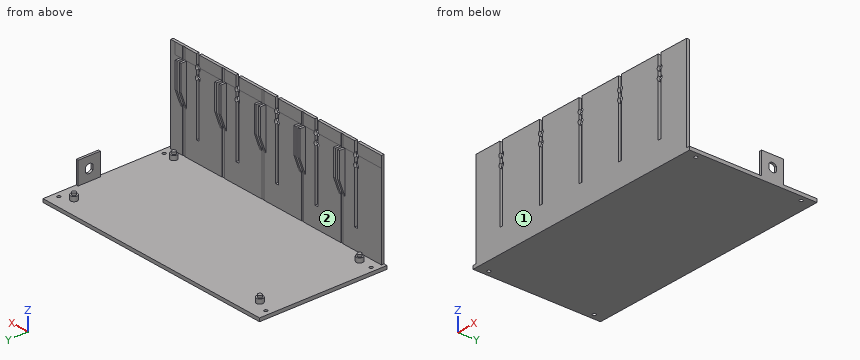
from build123d import *

# Parameters (mm, degrees)
SKETCH_W        = 226
SKETCH_H        = 115
PAD_DEPTH       = 3
PAD001_DEPTH    = 85
SKETCH002_R     = 3
PAD002_DEPTH    = 4
SKETCH003_R     = 1.75
PAD003_DEPTH    = 2
SKETCH004_R     = 1.5
POCKET_DEPTH    = 3.001
SKETCH005_W     = 3
SKETCH005_H     = 10.331698
SKETCH005_H_2   = 9.573412
SKETCH005_H_3   = 9.002111
SKETCH005_H_4   = 9.234924
SKETCH005_H_5   = 9.778156
POCKET001_DEPTH = 67
SKETCH006_R     = 2.5
POCKET002_DEPTH = 5
SKETCH008_W     = 218.676559
SKETCH008_H     = 5.389001
POCKET003_DEPTH = 10
POCKET004_DEPTH = 200
SKETCH010_W     = 2
SKETCH010_H     = 20
PAD004_DEPTH    = 20
POCKET005_DEPTH = 5
SKETCH012_W     = 3
SKETCH012_H     = 3
POCKET006_DEPTH = 85


with BuildPart() as part:
    # Sketch → Pad (new body)
    with BuildSketch(Plane.XY):
        with Locations((113, 57.5)):
            Rectangle(SKETCH_W, SKETCH_H)
    extrude(amount=PAD_DEPTH)

    # Sketch001 (on Face6 of Pad) → Pad001 (join)
    with BuildSketch(Plane.XY.offset(3)):
        Polygon((0, 0), (0, 2.4), (41.05, 2.4), (41.05, 7.4), (43.05, 7.4), (43.05, 2), (45.35, 2), (45.35, 7.4), (47.35, 7.4), (47.35, 2.4), (82.35, 2.4), (82.35, 7.4), (84.35, 7.4), (84.35, 2), (86.65, 2), (86.65, 7.4), (88.65, 7.4), (88.65, 2.4), (123.65, 2.4), (123.65, 7.4), (125.65, 7.4), (125.65, 2), (127.95, 2), (127.95, 7.4), (129.95, 7.4), (129.95, 2.4), (164.95, 2.4), (164.95, 7.4), (166.95, 7.4), (166.95, 2), (169.25, 2), (169.25, 7.4), (171.25, 7.4), (171.25, 2.4), (206.25, 2.4), (206.25, 7.4), (208.25, 7.4), (208.25, 2), (210.55, 2), (210.55, 7.4), (212.55, 7.4), (212.55, 2.4), (226, 2.4), (226, 0), align=None)
    extrude(amount=PAD001_DEPTH)

    # Sketch002 (on Face3 of Pad001) → Pad002 (join)
    with BuildSketch(Plane.XY.offset(3)):
        with Locations((17, 10)):
            Circle(SKETCH002_R)
        with Locations((17, 100)):
            Circle(SKETCH002_R)
        with Locations((211, 100)):
            Circle(SKETCH002_R)
        with Locations((211, 10)):
            Circle(SKETCH002_R)
    extrude(amount=PAD002_DEPTH)

    # Sketch003 (on Face54 of Pad002) → Pad003 (join)
    with BuildSketch(Plane.XY.offset(7)):
        with Locations((17, 100)):
            Circle(SKETCH003_R)
        with Locations((211, 100)):
            Circle(SKETCH003_R)
        with Locations((17, 10)):
            Circle(SKETCH003_R)
        with Locations((211, 10)):
            Circle(SKETCH003_R)
    extrude(amount=PAD003_DEPTH)

    # Sketch004 (on Face7 of Pad003) → Pocket (cut, through all)
    with BuildSketch(Plane.XY.offset(3)):
        with Locations((5, 105)):
            Circle(SKETCH004_R)
        with Locations((221, 105)):
            Circle(SKETCH004_R)
        with Locations((221, 10)):
            Circle(SKETCH004_R)
        with Locations((5, 10)):
            Circle(SKETCH004_R)
    extrude(amount=-POCKET_DEPTH, mode=Mode.SUBTRACT)

    # Sketch005 (on Face10 of Pocket) → Pocket001 (cut)
    with BuildSketch(Plane.XY.offset(88)):
        with Locations((29.55, 1.058323)):
            Rectangle(SKETCH005_W, SKETCH005_H)
        with Locations((70.85, 1.24642)):
            Rectangle(SKETCH005_W, SKETCH005_H_2)
        with Locations((112.15, 0.827586)):
            Rectangle(SKETCH005_W, SKETCH005_H_3)
        with Locations((153.45, 1.334431)):
            Rectangle(SKETCH005_W, SKETCH005_H_4)
        with Locations((194.75, 1.451644)):
            Rectangle(SKETCH005_W, SKETCH005_H_5)
    extrude(amount=-POCKET001_DEPTH, mode=Mode.SUBTRACT)

    # Sketch006 (on Face2 of Pocket001) → Pocket002 (cut)
    with BuildSketch(Plane.XZ):
        with Locations((29.55, 77)):
            Circle(SKETCH006_R)
        with Locations((29.55, 69)):
            Circle(SKETCH006_R)
        with Locations((70.85, 77)):
            Circle(SKETCH006_R)
        with Locations((70.85, 69)):
            Circle(SKETCH006_R)
        with Locations((112.15, 77)):
            Circle(SKETCH006_R)
        with Locations((112.15, 69)):
            Circle(SKETCH006_R)
        with Locations((153.45, 77)):
            Circle(SKETCH006_R)
        with Locations((153.45, 69)):
            Circle(SKETCH006_R)
        with Locations((194.75, 77)):
            Circle(SKETCH006_R)
        with Locations((194.75, 69)):
            Circle(SKETCH006_R)
    extrude(amount=-POCKET002_DEPTH, mode=Mode.SUBTRACT)

    # Sketch008 (on Face60 of Pocket002) → Pocket003 (cut)
    with BuildSketch(Plane.XY.offset(88)):
        with Locations((109.338279, 5.0945)):
            Rectangle(SKETCH008_W, SKETCH008_H)
    extrude(amount=-POCKET003_DEPTH, mode=Mode.SUBTRACT)

    # Sketch009 (on Face88 of Pocket003) → Pocket004 (cut)
    with BuildSketch(Plane.YZ.offset(212.55)):
        Polygon((7.4, 3), (2.4, 3), (2.4, 40.5), (7.4, 54.974999), align=None)
    extrude(amount=-POCKET004_DEPTH, mode=Mode.SUBTRACT)

    # Sketch010 (on Face132 of Pocket004) → Pad004 (join)
    with BuildSketch(Plane.XY.offset(3)):
        with Locations((225, 75)):
            Rectangle(SKETCH010_W, SKETCH010_H)
    extrude(amount=PAD004_DEPTH)

    # Sketch011 (on Face154 of Pad004) → Pocket005 (cut)
    with BuildSketch(Plane.YZ.offset(226)):
        with BuildLine():
            ThreePointArc((78.3, 15.085192), (75, 16.906731), (71.7, 15.085192))
            Line((71.7, 15.085192), (71.7, 10.92827))
            ThreePointArc((71.7, 10.92827), (75, 9.106731), (78.3, 10.92827))
            Line((78.3, 15.085192), (78.3, 10.92827))
        make_face()
    extrude(amount=-POCKET005_DEPTH, mode=Mode.SUBTRACT)

    # Sketch012 (on Face80 of Pocket005) → Pocket006 (cut)
    with BuildSketch(Plane.XY.offset(88)):
        with Locations((1.5, 1.5)):
            Rectangle(SKETCH012_W, SKETCH012_H)
        with Locations((224.5, 1.5)):
            Rectangle(SKETCH012_W, SKETCH012_H)
    extrude(amount=-POCKET006_DEPTH, mode=Mode.SUBTRACT)


solid = part.part
The listing builds one solid part. Answer for the finished solid, in the listing's coordinates (mm). Face numbers are marked on the shaded views. Coordinates: 2 decimals unless noted, no trailing zeros. Order: outer loops, then holes, each group sorted by start corner. A loop starts at its lowest first (then second) coordinate and runs counter-clockwise, first axis right, second up. Notation, with made-up numbers: M 37,58.25 L 78,58.25 A17 ccw 78,87.25 Z; hole C 79.25,30 d5. An arc over 180 degrees is marked long. Use CSV: the item, a comma, the result in double quotes.
Q1. Determine the mould class of the marked faces 1 and 2 for opening direction X: pulls with the +X half, pulls with the -X half, needs draft (parallel to the pull), parting line crosses it, or undercut.
Here are the results:
face 1,"needs draft"
face 2,"undercut"
Q2. Given pin 1 Ø0.7 at (y, z) = (1, 84) entering from -X; pin 2 Ø1.2 at (y, z) = (1.5, 74) entering from +X; pin 3 Ø1 at (x, z) = (83.5, 65) entering from +Y; pin 4 Ø4.5 at (y, z) = (5, 31.5) entering from -X, each flat-ended and moving along its own axis, determine where each tip first touches the part or whether it passes through.
Here are the results:
pin 1,"x = 3"
pin 2,"x = 223"
pin 3,"y = 7.4"
pin 4,"through"
Q3. Section C-C (y = 57) is taken. Determine the outline of the cut face in (x, z), then the cut area to 3 significant figures.
Here are the results:
outline,"M 0,0 L 226,0 L 226,3 L 0,3 Z"
area,"678 mm2"
Q4. Section B-B (z = 63.5) is taken. Give the number of separate pieces and of enclosed holes in the cut face, then the cut area to 3 significant figures.
Here are the results:
separate pieces,"6"
enclosed holes,"0"
area,"587 mm2"
Q5. Section A-A (x = 203) is taken. Determine the outline of the cut face in (y, z), then the cut area to 3 significant figures.
Here are the results:
outline,"M 0,0 L 115,0 L 115,3 L 2.4,3 L 2.4,88 L 0,88 Z"
area,"549 mm2"
Q6. Straight lines are drawn through the part: L1, parallel to Y at x = 221, z = 1.6; L2, parallel to X at y = 105, z = 1.55; L3, parallel to Z at x = 196.5, y = 65. For each, find the intervals that lie inside material, in ascending order.
Here are the results:
L1,"0 to 8.5, 11.5 to 103.5, 106.5 to 115"
L2,"0 to 3.5, 6.5 to 219.5, 222.5 to 226"
L3,"0 to 3"
